from build123d import *

# Parameters (mm, degrees)
SKETCH_1_R               = 3
EXTRUDE_1_DEPTH          = 27
CUT_EXTRUDE_1_DEPTH      = 0.35
CUT_EXTRUDE_1_DEPTH_BACK = 0.35
SKETCH_2_R               = 3
SKETCH_2_R_2             = 2.75
CUT_EXTRUDE_START        = -0.7
SKETCH_3_R               = 3
SKETCH_3_R_2             = 2.75
CUT_EXTRUDE_2_DEPTH      = 0.7


with BuildPart() as part:
    # 스케치1 → 보스-돌출1 (new body)
    with BuildSketch(Plane.XY):
        Circle(SKETCH_1_R)
    extrude(amount=EXTRUDE_1_DEPTH)

    # 스케치2 → 컷-돌출1 (cut, two sides: drawn at the far end of the back side and taken through both)
    with BuildSketch(Plane.XY.offset(25.5).offset(-CUT_EXTRUDE_1_DEPTH_BACK)):
        Circle(SKETCH_2_R)
        Circle(SKETCH_2_R_2, mode=Mode.SUBTRACT)
    extrude(amount=CUT_EXTRUDE_1_DEPTH + CUT_EXTRUDE_1_DEPTH_BACK, mode=Mode.SUBTRACT)

    # 스케치3 → 컷-돌출2 (cut)
    with BuildSketch(Plane.XY.offset(15.15).offset(CUT_EXTRUDE_START)):
        Circle(SKETCH_3_R)
        Circle(SKETCH_3_R_2, mode=Mode.SUBTRACT)
    extrude(amount=CUT_EXTRUDE_2_DEPTH, mode=Mode.SUBTRACT)


solid = part.part
For this review, take the finished solid that the model builds, in its own axes (mm). A direction names the side the tool comes from. Coordinates: 2 decimals unless noted, no trailing zeros. Write each loop counter-clockwise with the first axis right and the second up, starting at its lowest first coordinate (ties: lowest second). Pieces come first, ordered by that corner, then holes. Notation, with made-up numbers: (-1.75, -33) -> (23.25, -33) arc R22 ccw to (23.25, -18) -> close; hole circle Ø2 at (53, -16.75). An arc over 180 degrees is marked (long way). Write each question's results on one line, items separated by ' | '. Start each with the question number.
1) The part is to be moulded in two halves that separate along Z. For faces 3 (the face through (-3, 0, 26)), 4 (the face through (0, 0, 0)), 5 (the face through (-0.596, -2.685, 14.795)), say which applies: +Z half, -Z half, draft (parallel to the pull), parting line (faces both ways), or undercut.
2) Consider section A-A (x = -1.9). Write out the cut boundary in (y, z).
3) Consider section B-B (y = -2.3). Write out the cut boundary in (x, z).
4) Wall thickness on L1, parallel to Z at x = 1.9, y = -2.2; L2, parallel to Y at x = 0.15, z = 15.75; L3, parallel to Y at x = -2.45, z = 14: over which ranges is each line inside the solid? List them lowest first. Write a range as [from, to].
5) Insertion check: pin 1 (1.5 mm diameter, centred on y = -1.5, z = 23.5, fed in from +X). The pin has a flat end and moves straight along its axis. Give the tip position at first contact, or say it passes through.
6) Consider section C-C (z = 22.75). Write out the cut boundary in (x, y), plus the area to 3 significant figures.
7) For faces 1 (the face through (-0.596, -2.685, 25.495)), 2 (the face through (-3, 0, 20)), list the 3-axis set-ups (+Z, -Z, +X, -X, +Y, -Y) from which the entire face can be reached by the end or side of a thin tool; tool diameter is ignored.
Geometry says:
1) face 3: draft | face 4: -Z half | face 5: undercut
2) outline: (-2.32, 0) -> (2.32, 0) -> (2.32, 14.45) -> (1.99, 14.45) -> (1.99, 15.15) -> (2.32, 15.15) -> (2.32, 25.15) -> (1.99, 25.15) -> (1.99, 25.85) -> (2.32, 25.85) -> (2.32, 27) -> (-2.32, 27) -> (-2.32, 25.85) -> (-1.99, 25.85) -> (-1.99, 25.15) -> (-2.32, 25.15) -> (-2.32, 15.15) -> (-1.99, 15.15) -> (-1.99, 14.45) -> (-2.32, 14.45) -> close
3) outline: (-1.93, 0) -> (1.93, 0) -> (1.93, 14.45) -> (1.51, 14.45) -> (1.51, 15.15) -> (1.93, 15.15) -> (1.93, 25.15) -> (1.51, 25.15) -> (1.51, 25.85) -> (1.93, 25.85) -> (1.93, 27) -> (-1.93, 27) -> (-1.93, 25.85) -> (-1.51, 25.85) -> (-1.51, 25.15) -> (-1.93, 25.15) -> (-1.93, 15.15) -> (-1.51, 15.15) -> (-1.51, 14.45) -> (-1.93, 14.45) -> close
4) L1: [0, 14.45], [15.15, 25.15], [25.85, 27] | L2: [-3, 3] | L3: [-1.73, 1.73]
5) pin 1: x = 2.9
6) outline: circle Ø6 at (0, 0) | area: 28.3 mm^2
7) face 1: none | face 2: +Z, -Z
